Answer from the drawing. Dimensions are ordinates in mm from the lowest x, y and z of the part. Coordinates: 2 decimals unless noted, no trailing zeros. Write each loop counter-clockwise with the first axis right and the second up, starting at its lowest first coordinate (ties: lowest second). Pieces come first, ordered by that corner, then holes. Notation, with made-up numbers: (20, -19.5) - (55, -19.5) arc R21 cw to (55, -6.5) - close; hole circle Ø10 at (1.5, 27.25). An arc over 180 degrees is marked (long way). Use one line per item in the form item = value. Start each with the question number.
Item 1: Given pin 1 (1 mm diameter, centred on x = 75.5, z = 2.5, fed in from +Y); pin 2 (1.5 mm diameter, centred on x = 25, z = 2.5, fed in from +Y) (1 decimal); pin 3 (1.5 mm diameter, centred on y = 75.5, z = 2.5, fed in from +X), each flat-ended and moving along its own axis, determine where each tip first touches the part or whether it passes through.
Item 2: A cutting plane is placed at A-A (x = 44.45). Write down the section's boundary in (y, z).
Item 3: Consider probe 1 along X at (y, z) = (45, 5); probe 2 along X at (y, z) = (57.5, 5) (1 decimal); probe 3 along Y at (x, z) = (46, 3.25). Determine where each line is inside the solid, lowest interval first.
Item 4: Determine the mould class of the marked faces 1, 2 and 3 for opening direction Y: released by +Y, released by -Y, zero draft, split by the parting line, or undercut.
Item 5: A cutting plane is placed at C-C (z = 2.5). Give the number of separate pieces and of enclosed holes in the cut face, then the cut area to 3 significant figures.
Item 6: A cutting plane is placed at D-D (x = 79). Write down the section's boundary in (y, z), then the cut area to 3 significant figures.
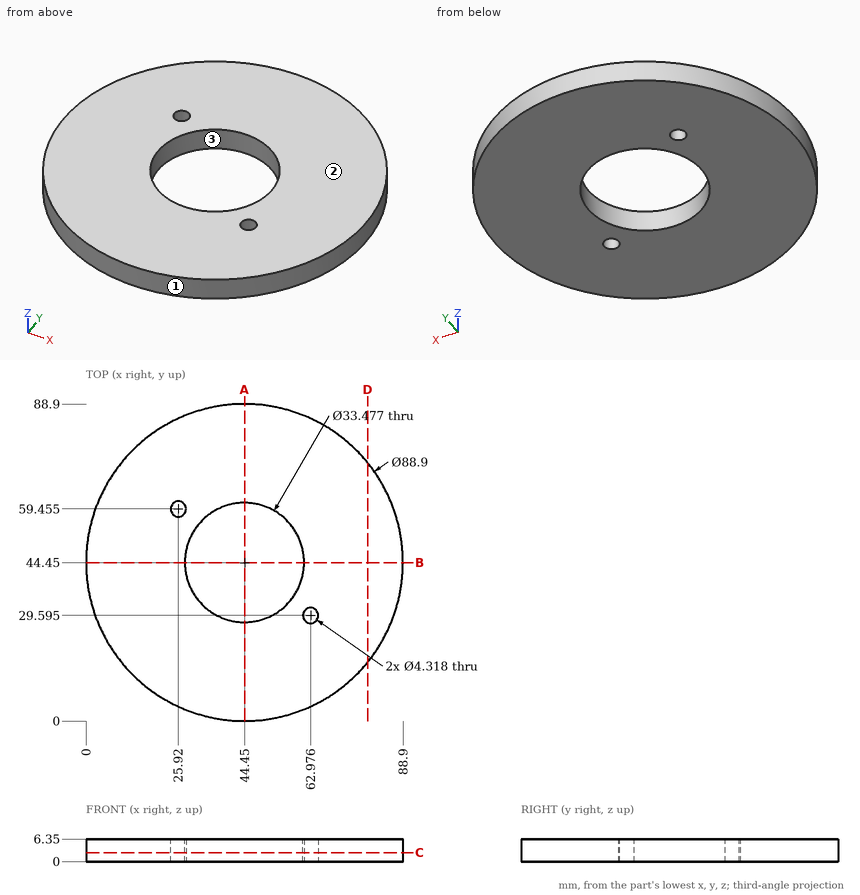
Answer:
q1.pin_1 = 76.74
q1.pin_2 = 84.8
q1.pin_3 = 76.97
q2.outline = (0, 0) - (27.71, 0) - (27.71, 6.35) - (0, 6.35) - close; (61.19, 0) - (88.9, 0) - (88.9, 6.35) - (61.19, 6.35) - close
q3.probe_1 = 0 to 27.72, 61.18 to 88.9
q3.probe_2 = 2 to 25, 26.8 to 34, 54.9 to 86.9
q3.probe_3 = 0.03 to 27.78, 61.12 to 88.87
q4.face_1 = split by the parting line
q4.face_2 = zero draft
q4.face_3 = undercut
q5.separate_pieces = 1
q5.enclosed_holes = 3
q5.area = 5,300 mm²
q6.outline = (16.48, 0) - (72.42, 0) - (72.42, 6.35) - (16.48, 6.35) - close
q6.area = 355 mm²
